Could you check a few things on this model? Use its own coordinates, in mm. A direction names the side the tool comes from. Coordinates: 2 decimals unless noted, no trailing zeros. Write each loop counter-clockwise with the first axis right and the second up, starting at its lowest first coordinate (ties: lowest second). Pieces come first, ordered by that corner, then holes.
Item 1: Which directions (+Z, -Z, +X, -X, +Y, -Y) give clear straight access to the entire face, cutting with the end or side of a thin tool? Please do faces 5 (the flat face through (-13, 14, 3)), 6 (the flat face through (37.25, 14, 8)).
Item 2: For P1, Ø10.5, axis at x = 22.5, z = -6.5, coming from the +Y side; P2, Ø5, axis at x = -14.5, y = 16, coming from the +Z side; P3, Ø4, axis at y = 13.5, z = -16.5, coming from the +X side, each with a flat end and sliding along its axis, tell me the tip position at first contact or that it passes through.
Item 3: If I drill on probe 1 along X at (y, z) = (30, 0); probe 2 along X at (y, z) = (16, -5) (3 decimals); probe 3 along Y at (x, z) = (-43.5, 36.5), over which ranges is the centre line in solid material (lowest first)?
Item 4: I want a section at C-C on x = 0. Please give me the cut outline in (y, z), then the cut area to 3 significant figures.
Item 5: I want a section at B-B on y = 25. Please give me the cut outline in (x, z) (3 decimals).
Item 6: Thinking about a two-plate mould opening in Y: for faces 1 (the flat face through (1, -3, -1)), 2 (the flat face through (-64, 14, -3)), 3 (the flat face through (-16.75, 14, 8)), 4 (the flat face through (64, 28.65, 0)), which applies, +Y half, -Y half, draft (parallel to the pull), parting line (faces both ways), or undercut?
Item 7: I want a section at A-A on z = 0. Please give me the cut outline in (x, y).
Item 8: I want a section at D-D on z = 47.5. Please give me the cut outline in (x, y), then the cut area to 3 significant figures.
from build123d import *

# Parameters (mm, degrees)
SKETCH1_R               = 66.5
SKETCH1_R_2             = 62.5
BOSS_EXTRUDE1_DEPTH     = 46.8
SKETCH1_3_R             = 75
SKETCH1_3_R_2           = 66.5
BOSS_EXTRUDE2_DEPTH     = 3
BOSS_EXTRUDE3_START     = -3
SKETCH1_5_R             = 66.5
SKETCH1_5_R_2           = 62.5
BOSS_EXTRUDE3_DEPTH     = 3
SKETCH2_W               = 54
SKETCH2_H               = 25
SKETCH2_R               = 0.875
SKETCH2_W_2             = 41
SKETCH2_H_2             = 21
BOSS_EXTRUDE4_DEPTH     = 28.65
CUT_EXTRUDE1_DEPTH      = 128.409978024
CUT_EXTRUDE1_DEPTH_BACK = 128.409978024
SKETCH3_W               = 3
SKETCH3_H               = 28.65


with BuildPart() as part:
    # Sketch1 → Boss-Extrude1 (new body)
    with BuildSketch(Plane(origin=(0, 0, 0), x_dir=(1, 0, 0), z_dir=(0, 1, 0))):
        with Locations(Location((0, 0, 0), (0, 0, 270))):
            Circle(SKETCH1_R)
        with Locations(Location((0, 0, 0), (0, 0, 270))):
            Circle(SKETCH1_R_2, mode=Mode.SUBTRACT)
    extrude(amount=BOSS_EXTRUDE1_DEPTH)



with BuildPart() as body_2:
    # Sketch1_3 → Boss-Extrude2 (new body)
    with BuildSketch(Plane(origin=(0, 0, 0), x_dir=(1, 0, 0), z_dir=(0, 1, 0))):
        with Locations(Location((0, 0, 0), (0, 0, 270))):
            Circle(SKETCH1_3_R)
        with Locations(Location((0, 0, 0), (0, 0, 270))):
            Circle(SKETCH1_3_R_2, mode=Mode.SUBTRACT)
    extrude(amount=-BOSS_EXTRUDE2_DEPTH)


with BuildPart() as part_1:
    add(part.part)

    add(body_2.part)  # Boss-Extrude3 merges body 2
    # Sketch1_5 → Boss-Extrude3 (add)
    # profile 1 of 2: a face of its own
    with BuildSketch(Plane(origin=(0, 0, 0), x_dir=(1, 0, 0), z_dir=(0, 1, 0)).offset(BOSS_EXTRUDE3_START)):
        with Locations(Location((0, 0, 0), (0, 0, 270))):
            Circle(SKETCH1_5_R)
        with Locations(Location((0, 0, 0), (0, 0, 270))):
            Circle(SKETCH1_5_R_2, mode=Mode.SUBTRACT)
    # profile 2 of 2: a face of its own
    with BuildSketch(Plane(origin=(0, 0, 0), x_dir=(1, 0, 0), z_dir=(0, 1, 0)).offset(BOSS_EXTRUDE3_START)):
        with Locations(Location((0, 0, 0), (0, 0, 270))):
            Circle(SKETCH1_5_R_2)
    extrude(amount=BOSS_EXTRUDE3_DEPTH)

    # Sketch2 → Boss-Extrude4 (add)
    with BuildSketch(Plane(origin=(0, 0, 0), x_dir=(1, 0, 0), z_dir=(0, 1, 0))):
        with Locations((10.25, 0)):
            Rectangle(SKETCH2_W, SKETCH2_H)
        with Locations(Location((-13.75, -5, 0), (0, 0, 270))):
            Circle(SKETCH2_R, mode=Mode.SUBTRACT)
        with Locations(Location((-13.75, 5, 0), (0, 0, 270))):
            Circle(SKETCH2_R, mode=Mode.SUBTRACT)
        with Locations(Location((34.25, 5, 0), (0, 0, 270))):
            Circle(SKETCH2_R, mode=Mode.SUBTRACT)
        with Locations(Location((34.25, -5, 0), (0, 0, 270))):
            Circle(SKETCH2_R, mode=Mode.SUBTRACT)
        with Locations((10.25, 0)):
            Rectangle(SKETCH2_W_2, SKETCH2_H_2, mode=Mode.SUBTRACT)
    extrude(amount=BOSS_EXTRUDE4_DEPTH)

    # Sketch3 → Cut-Extrude1 (cut, two sides: drawn at the far end of the back side and taken through both)
    with BuildSketch(Plane.ZY.offset(16.75).offset(-CUT_EXTRUDE1_DEPTH_BACK)):
        with Locations((1.5, 14.325)):
            Rectangle(SKETCH3_W, SKETCH3_H)
        with Locations((-1.5, 14.325)):
            Rectangle(SKETCH3_W, SKETCH3_H)
    extrude(amount=CUT_EXTRUDE1_DEPTH + CUT_EXTRUDE1_DEPTH_BACK, mode=Mode.SUBTRACT)


solid = part_1.part
Response values:
1. face 5: +X, -X, +Y
1. face 6: +Y
2. P1: stops at y = 28.65
2. P2: stops at z = 65.41
2. P3: stops at x = 64.9
3. probe 1: x = -66.5 to -62.5, 62.5 to 66.5
3. probe 2: x = -66.312 to -62.3, -16.75 to -14.625, -12.875 to -10.25, 30.75 to 33.375, 35.125 to 37.25, 62.3 to 66.312
3. probe 3: y = -3 to 0
4. outline: (-3, -75) - (0, -75) - (0, -66.5) - (46.8, -66.5) - (46.8, -62.5) - (0, -62.5) - (0, -12.5) - (28.65, -12.5) - (28.65, -10.5) - (0, -10.5) - (0, 10.5) - (28.65, 10.5) - (28.65, 12.5) - (0, 12.5) - (0, 62.5) - (46.8, 62.5) - (46.8, 66.5) - (0, 66.5) - (0, 75) - (-3, 75) - close
4. area: 939 mm2
5. outline: (-66.432, -3) arc R66.5 ccw to (66.432, -3) - (62.428, -3) arc R62.5 cw to (-62.428, -3) - close; (-66.432, 3) - (-62.428, 3) arc R62.5 cw to (62.428, 3) - (66.432, 3) arc R66.5 ccw to start; (-16.75, -12.5) - (37.25, -12.5) - (37.25, -3) - (30.75, -3) - (30.75, -10.5) - (-10.25, -10.5) - (-10.25, -3) - (-16.75, -3) - close; (-16.75, 3) - (-10.25, 3) - (-10.25, 10.5) - (30.75, 10.5) - (30.75, 3) - (37.25, 3) - (37.25, 12.5) - (-16.75, 12.5) - close; hole circle Ø1.75 at (-13.75, -5); hole circle Ø1.75 at (-13.75, 5); hole circle Ø1.75 at (34.25, -5); hole circle Ø1.75 at (34.25, 5)
6. face 1: -Y half
6. face 2: undercut
6. face 3: draft
6. face 4: undercut
7. outline: (-75, -3) - (75, -3) - (75, 0) - (-75, 0) - close; (-66.5, 28.65) - (-62.5, 28.65) - (-62.5, 46.8) - (-66.5, 46.8) - close; (62.5, 28.65) - (66.5, 28.65) - (66.5, 46.8) - (62.5, 46.8) - close
8. outline: (-58.04, -3) - (58.04, -3) - (58.04, 0) - (46.54, 0) - (46.54, 46.8) - (40.62, 46.8) - (40.62, 0) - (-40.62, 0) - (-40.62, 46.8) - (-46.54, 46.8) - (-46.54, 0) - (-58.04, 0) - close
8. area: 902 mm2
